Design review of the part built by this model. Coordinates are the model's own, in mm. Face numbers are marked on the shaded views. A direction names the side the tool comes from. Coordinates: 2 decimals unless noted, no trailing zeros. Loops run counter-clockwise (first coordinate to the right, second up) from the corner with the lowest first, then second, coordinate; pieces in that order, holes last. Notation, with made-up numbers: (87.5, 85) -> (122.5, 85) arc R24 cw to (122.5, 115) -> close; hole circle Ø10 at (50.25, 27). An arc over 180 degrees is marked (long way). Use one line per item in the form item = value. Start each with the question number.
1. Consider section D-D (y = 10.75). State the section outline as (x, z) points.
2. Machinability: for the marked faces 1 and 2, which of the approach directions +Z, -Z, +X, -X, +Y, -Y give a long, thin tool a straight path to every point of the face, cutting with its end or side? Answer none if there is none.
3. Consider section C-C (z = 2.5). State the section outline as (x, y) points, then the cut area to 3 significant figures.
4. Consider section A-A (y = 1). State the section outline as (x, z) points.
5. Wall thickness on line 1 (X direction, y = 3, z = 4.75); line 2 (Z direction, x = -2.75, y = 2.75); line 3 (Y direction, x = -4.75, z = 1.5): over which ranges is each line inside the solid? List them lowest first. Write a range as from..to.
6. The part is to be moulded in two halves that separate along X. For the marked faces 3, 4 and 5, say which applies: released by +X, released by -X, zero draft, split by the parting line, or undercut.
7. For pin 1 (2 mm diameter, centred on x = -2, z = -0.5, fed in from -Y), flat-tipped, find the tip position at first contact; note if it passes through.
8. Consider section B-B (x = -3.25). State the section outline as (y, z) points.
from build123d import *

# Parameters (mm, degrees)
F1_DEPTH = 2.5
F0_W     = 4
F0_H     = 10
F2_DEPTH = 2
F5_R     = 2


with BuildPart() as f1:
    # F0 (on Top) → F1 (new body)
    with BuildSketch(Plane.XY):
        Polygon((0, 12), (0, 0), (1, 0), (1, 10), (5, 10), (5, 0), (7, 0), (7, 12), align=None)
    extrude(amount=F1_DEPTH)

    # F0 (on Top) → F2 (join)
    with BuildSketch(Plane.XY):
        with Locations((3, 5)):
            Rectangle(F0_W, F0_H)
        Polygon((0, 12), (0, 0), (1, 0), (1, 10), (5, 10), (5, 0), (7, 0), (7, 12), align=None)
    extrude(amount=-F2_DEPTH)

    # F3: F1 across face


with BuildPart() as f1_1:
    add(f1.part)
    add(f1.part.mirror(Plane(origin=(0, 6, 0.25), x_dir=(0, -1, 0), z_dir=(-1, 0, 0))))

    # F4: F1 across face


with BuildPart() as f1_2:
    add(f1_1.part)
    add(f1_1.part.mirror(Plane(origin=(0, 6.9090909091, 2.5), x_dir=(1, 0, 0), z_dir=(0, 0, 1))))

    # F5
    f5_edges = [f1_2.edges().sort_by_distance(p)[0] for p in [
        (0, 12, 7),
        (7, 12, 2.5),
        (0, 12, -2),
        (-7, 12, 2.5),
        (7, 6, 7),
        (-7, 6, 7),
        (7, 6, -2),
        (-7, 6, -2),
    ]]
    fillet(f5_edges, radius=F5_R)


solid = f1_2.part
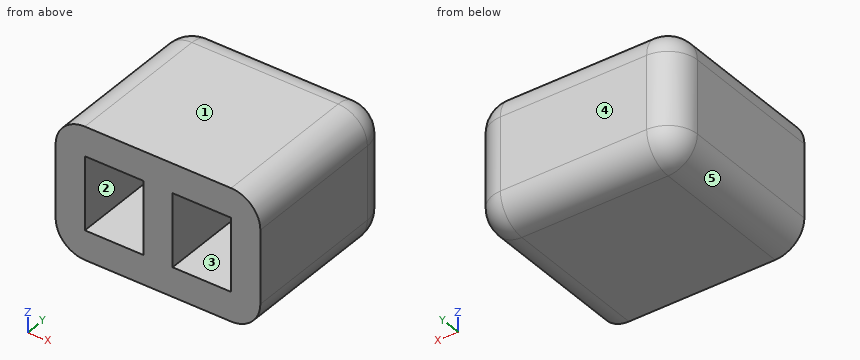
Geometry check:
q1.outline = (-6.85, 0) arc R1.85 ccw to (-5, -1.85) -> (5, -1.85) arc R1.85 ccw to (6.85, 0) -> (6.85, 5) arc R1.85 ccw to (5, 6.85) -> (-5, 6.85) arc R1.85 ccw to (-6.85, 5) -> close
q2.face_1 = +Z, +X, -X, +Y, -Y
q2.face_2 = -Y
q3.outline = (-7, 0) -> (-5, 0) -> (-5, 10) -> (-1, 10) -> (-1, 0) -> (1, 0) -> (1, 10) -> (5, 10) -> (5, 0) -> (7, 0) -> (7, 10) arc R2 ccw to (5, 12) -> (-5, 12) arc R2 ccw to (-7, 10) -> close
q3.area = 86.3 mm²
q4.outline = (-7, 0) arc R2 ccw to (-5, -2) -> (5, -2) arc R2 ccw to (7, 0) -> (7, 5) arc R2 ccw to (5, 7) -> (-5, 7) arc R2 ccw to (-7, 5) -> close; hole (-5, 0) -> (-1, 0) -> (-1, 5) -> (-5, 5) -> close; hole (1, 0) -> (5, 0) -> (5, 5) -> (1, 5) -> close
q5.line_1 = -7..-5, -1..1, 5..7
q5.line_2 = -2..0, 5..7
q5.line_3 = 10..12
q6.face_3 = undercut
q6.face_4 = zero draft
q6.face_5 = released by -X
q7.pin_1 = 0
q8.outline = (0, -2) -> (10, -2) arc R2 ccw to (12, 0) -> (12, 5) arc R2 ccw to (10, 7) -> (0, 7) -> (0, 5) -> (10, 5) -> (10, 0) -> (0, 0) -> close
